```python
from build123d import *

# Parameters (mm, degrees)
F0_W     = 19.05
F0_H     = 166.624
F1_DEPTH = 252.4125
F3_W     = 19.05
F3_H     = 20.828
F4_DEPTH = 19.051
F7_R     = 101.6
F8_DEPTH = 10.4902


# Not quite as in the source:
# - a length typed as a fraction of an inch, garbled in the dataset ("3 / 203.2 mm" for 3/8 in), is restored


with BuildPart() as f1:
    # F0 (on Front) → F1 (new body)
    with BuildSketch(Plane.XZ):
        with Locations((-9.525, 83.312)):
            Rectangle(F0_W, F0_H)
    extrude(amount=-F1_DEPTH)

    # F3 (on Right) → F4 (cut, through all)
    with BuildSketch(Plane.YZ):
        with Locations((9.525, 135.382)):
            Rectangle(F3_W, F3_H)
        with Locations((9.525, 93.726)):
            Rectangle(F3_W, F3_H)
        with Locations((9.525, 52.07)):
            Rectangle(F3_W, F3_H)
        with Locations((9.525, 10.414)):
            Rectangle(F3_W, F3_H)
    extrude(amount=-F4_DEPTH, mode=Mode.SUBTRACT)

    # F5: F1 across face


with BuildPart() as f1_1:
    add(f1.part)
    add(f1.part.mirror(Plane(origin=(-9.525, 252.4125, 83.312), x_dir=(1, 0, 0), z_dir=(0, 1, 0))))

    # F7 (on offset) → F8 (cut, symmetric)
    with BuildSketch(Plane.XY.offset(76.2)):
        with Locations((-111.125, 252.4125)):
            Circle(F7_R)
    extrude(amount=F8_DEPTH, both=True, mode=Mode.SUBTRACT)


solid = f1_1.part
```
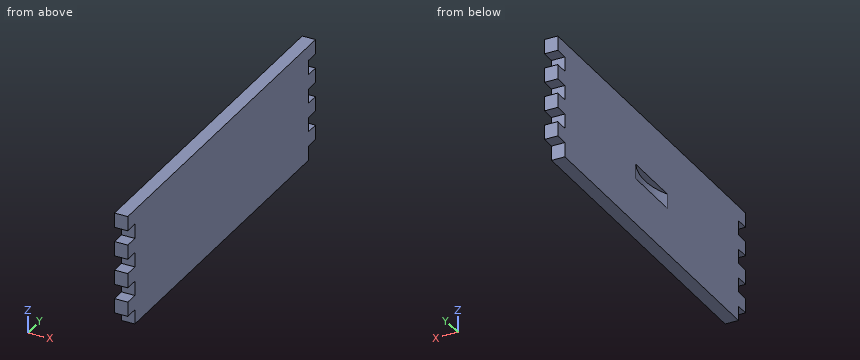
Geometry: final body of the model. Coordinates: model frame, mm. Give positions to 0.01 mm unless a question says otherwise; leave off trailing zeros. Write each loop counter-clockwise with the first axis right and the second up, starting at its lowest first coordinate (ties: lowest second). Pieces come first, ordered by that corner, then holes.
1. Pin query (flat end, axial travel): P1, Ø9.5, axis at x = -7, y = 499.5, coming from the -Z side; P2, Ø9.5, axis at x = -11, z = 96, coming from the -Y side. Return the tip coordinate at first contact, or that it passes through.
2. Section query C-C, the plane y = 259.5. Return loops of the section in (x, z), then the cut area to 3 significant figures.
3. Line query: probe 1 along Z at (x, y) = (-16, 227.5); probe 2 along Y at (x, z) = (-6.75, 133) (3 decimals). Output: solid intervals per line, ascending.
4. Section query B-B, the plane z = 16. Return loops of the section in (x, y) (3 decimals), then the cut area to 3 significant figures.
Computed:
1. P1: stops at z = 20.83
1. P2: stops at y = 19.05
2. outline: (-19.05, 0) - (0, 0) - (0, 166.62) - (-19.05, 166.62) - (-19.05, 86.69) - (-9.77, 86.69) - (-9.77, 65.71) - (-19.05, 65.71) - close
2. area: 2,980 mm2
3. probe 1: z = 0 to 65.71, 86.69 to 166.62
3. probe 2: y = 19.05 to 485.775
4. outline: (-19.05, 19.05) - (0, 19.05) - (0, 485.775) - (-19.05, 485.775) - close
4. area: 8,890 mm2
